Could you check a few things on this model? Use its own coordinates, in mm. A direction names the side the tool comes from. Coordinates: 2 decimals unless noted, no trailing zeros. Order: outer loops, then holes, each group sorted by start corner. A loop starts at its lowest first (then second) coordinate and runs counter-clockwise, first axis right, second up. Notation, with made-up numbers: (21.25, 50.25) - (32.25, 50.25) arc R26 cw to (32.25, 65.25) - close; hole circle Ø3 at (71, 33.5). An arc over 180 degrees is marked (long way). One line per item, written item: value. Start each with the question number.
from build123d import *

# Parameters (mm, degrees)
SKETCH1_R           = 17.5
BOSS_EXTRUDE1_DEPTH = 1.5
SKETCH2_R           = 40
BOSS_EXTRUDE2_DEPTH = 6.5
SKETCH3_W           = 250
SKETCH3_H           = 500
BOSS_EXTRUDE3_DEPTH = 20
FILLET2_R           = 1


with BuildPart() as part:
    # Sketch1 → Boss-Extrude1 (new body)
    with BuildSketch(Plane.XY):
        Circle(SKETCH1_R)
    extrude(amount=BOSS_EXTRUDE1_DEPTH)

    # Sketch2 → Boss-Extrude2 (add)
    with BuildSketch(Plane.XY.offset(1.5)):
        with Locations(Location((0, 0, 0), (0, 0, 180))):
            Circle(SKETCH2_R)
    extrude(amount=BOSS_EXTRUDE2_DEPTH)

    # Sketch3 → Boss-Extrude3 (add)
    with BuildSketch(Plane.XY.offset(8)):
        Rectangle(SKETCH3_W, SKETCH3_H)
    extrude(amount=BOSS_EXTRUDE3_DEPTH)

    # Fillet2
    fillet2_edges = [part.edges().sort_by_distance(p)[0] for p in [
        (40, 0, 8),
    ]]
    fillet(fillet2_edges, radius=FILLET2_R)


solid = part.part
Q1. If I drill on L1, parallel to Z at x = -57, y = 132; L2, parallel to Z at x = 36, y = -9.5; L3, parallel to Y at x = -33, z = 3, over which ranges is the centre line in solid material (lowest first)?
Q2. I want a section at C-C on x = -68. Please give me the cut outline in (y, z).
Q3. Which directions (+Z, -Z, +X, -X, +Y, -Y) give clear straight access to the entire face, cutting with the end or side of a thin tool? Please do faces 1 (the flat face through (125, -3, 18)), 2 (the cylindrical face through (-13.887, -10.648, 0.74)).
Q4. I want a section at D-D on y = -102. Please give me the cut outline in (x, z).
Q5. I want a section at B-B on x = 0. Please give me the cut outline in (y, z), then the cut area to 3 significant figures.
Q6. I'm going to push flat-ended pins straight in: pin 1 (1 mm diameter, centred on x = 60.5, y = -15.5, fed in from -Z); pin 2 (3 mm diameter, centred on y = -189, z = 6, fed in from -X). Where does each tip first touch, or does it pass through?
Q7. I want a section at A-A on y = 0. Please give me the cut outline in (x, z).
Values follow:
1. L1: z = 8 to 28
1. L2: z = 1.5 to 28
1. L3: y = -22.61 to 22.61
2. outline: (-250, 8) - (250, 8) - (250, 28) - (-250, 28) - close
3. face 1: +Z, -Z, +X, +Y, -Y
3. face 2: -Z
4. outline: (-125, 8) - (125, 8) - (125, 28) - (-125, 28) - close
5. outline: (-250, 8) - (-41, 8) arc R1 cw to (-40, 7) - (-40, 1.5) - (-17.5, 1.5) - (-17.5, 0) - (17.5, 0) - (17.5, 1.5) - (40, 1.5) - (40, 7) arc R1 cw to (41, 8) - (250, 8) - (250, 28) - (-250, 28) - close
5. area: 10,600 mm^2
6. pin 1: stops at z = 8
6. pin 2: passes through
7. outline: (-125, 8) - (-41, 8) arc R1 cw to (-40, 7) - (-40, 1.5) - (-17.5, 1.5) - (-17.5, 0) - (17.5, 0) - (17.5, 1.5) - (40, 1.5) - (40, 7) arc R1 cw to (41, 8) - (125, 8) - (125, 28) - (-125, 28) - close
